Check sheet for the drawn part. Datum: minimum x, y, z corner. Units: mm. Coordinates: 2 decimals unless noted, no trailing zeros. Write each loop counter-clockwise with the first axis right and the second up, starting at its lowest first coordinate (ties: lowest second). Pieces come first, ordered by that corner, then holes. Notation, with made-up numbers: M -20,-32 L 37,-32 A30 cw 37,-10 Z; hole C 17.25,16.5 d7. An arc over 180 degrees is marked long. Answer as CSV lines item,"result". Start each with the question number.
Q1. Depth check by flat-ended pin: pin 1 Ø3 at (y, z) = (4.953, 4.953) entering from -X; pin 2 Ø5.5 at (y, z) = (4.5, 5.5) entering from +X. Enter the tip coordinate at first touch or a pass-through.
Q2. Thickness scan on line 1 along Y through (x, z) = (0.3, 5) (1 decimal); line 2 along X through (y, z) = (6.75, 2.5); line 3 along Z through (x, y) = (0.3, 7.75) (1 decimal). Record the ranges inside material, lowest first. Write a range as from..to.
Q3. Mould release check, pull along Z, two halves, no side actions. Record for the marked faces 1, 2 and 3: pulls with the +Z half, pulls with the -Z half, needs draft (parallel to the pull), parting line crosses it, or undercut.
Q4. Sectioned sample at D-D, the plane x = 0.4. Record the cut outline in (y, z) (1 decimal).
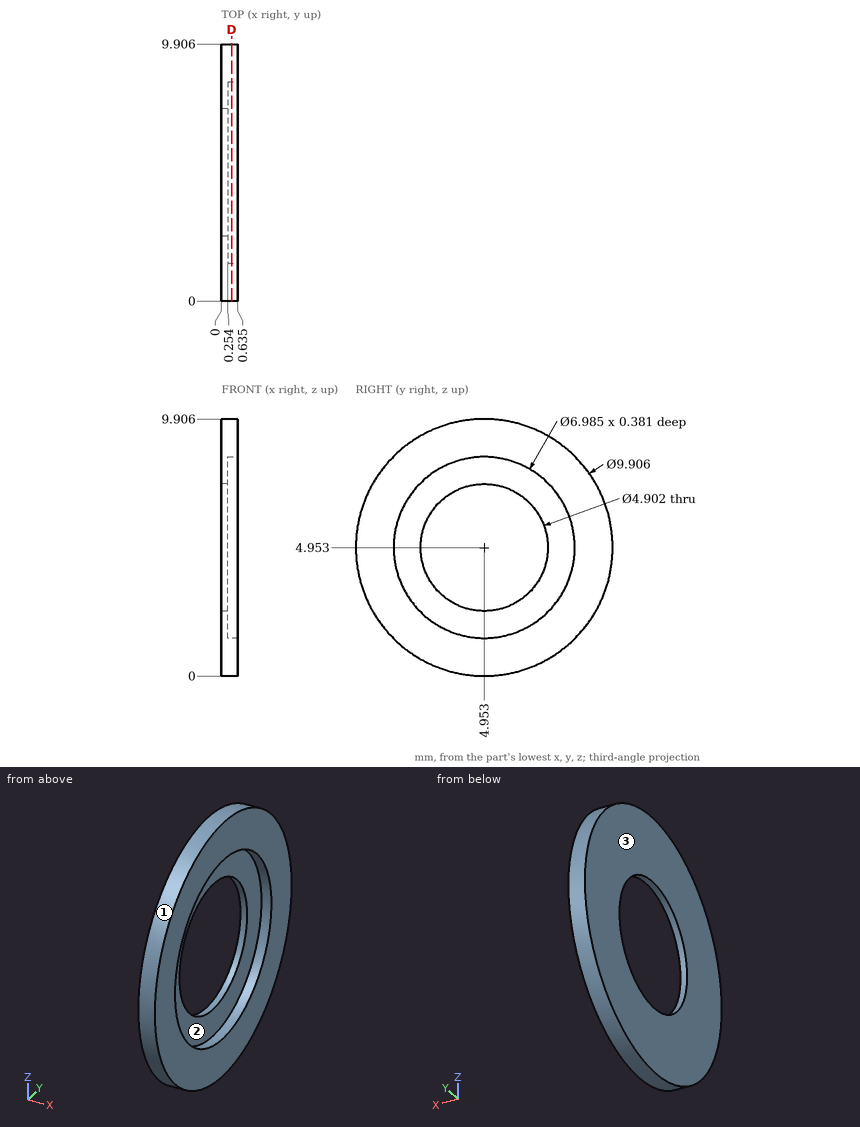
Output:
1,pin 1,"passes through"
1,pin 2,"stops at x = 0.25"
2,line 1,"y = 0..1.5, 8.4..9.9"
2,line 2,"x = 0..0.25"
2,line 3,"z = 0.9..2.9, 7..9"
3,face 1,"parting line crosses it"
3,face 2,"undercut"
3,face 3,"needs draft"
4,outline,"C 5,5 d9.9; hole C 5,5 d7"
